from build123d import *

# Parameters (mm, degrees)
F0_W      = 60.442928
F0_H      = 76.316834
F1_DEPTH  = 13
F2_R      = 4.501425
F3_DEPTH  = 7.874
F4_R      = 3.44672
F5_DEPTH  = 16.764
F6_W      = 10
F6_H      = 4.021608
F7_DEPTH  = 0.7
F8_W      = 12.088504
F8_H      = 2.308511
F9_DEPTH  = 7.874
F10_W     = 10
F10_H     = 2.673487
F11_DEPTH = 8.636
F12_W     = 10.518157
F12_H     = 2.767401
F13_DEPTH = 29.718
F14_R     = 1.567214
F15_DEPTH = 1
F16_W     = 1.627309
F16_H     = 5.575751
F17_DEPTH = 1


with BuildPart() as f1:
    # F0 (on Front) → F1 (new body)
    with BuildSketch(Plane.XZ):
        Rectangle(F0_W, F0_H)
    extrude(amount=F1_DEPTH)

    # F2 (on face) → F3 (cut)
    with BuildSketch(Plane(origin=(0, 0, 0), x_dir=(-1, 0, 0), z_dir=(0, 1, 0))):
        with Locations((-20.47102, 49.871981)):
            Circle(F2_R)
    extrude(amount=F3_DEPTH, mode=Mode.SUBTRACT)

    # F4 (on face) → F5 (cut)
    with BuildSketch(Plane.XY.offset(38.158417)):
        with Locations((22.332672, -8.926389)):
            Circle(F4_R)
    extrude(amount=-F5_DEPTH, mode=Mode.SUBTRACT)

    # F6 (on face) → F7 (join)
    with BuildSketch(Plane(origin=(0, 0, -38.158417), x_dir=(1, 0, 0), z_dir=(0, 0, -1))):
        with Locations((-17.087876, 8.49799)):
            Rectangle(F6_W, F6_H)
    extrude(amount=F7_DEPTH)

    # F8 (on face) → F9 (join)
    with BuildSketch(Plane.XY.offset(38.158417)):
        with Locations((0.475428, -10.475016)):
            Rectangle(F8_W, F8_H)
    extrude(amount=-F9_DEPTH)

    # F10 (on face) → F11 (join)
    with BuildSketch(Plane.XY.offset(38.158417)):
        with Locations((-1.288279, -8.985477)):
            Rectangle(F10_W, F10_H)
    extrude(amount=-F11_DEPTH)

    # F12 (on face) → F13 (cut)
    with BuildSketch(Plane.XY.offset(38.158417)):
        with Locations((0.831678, -10.416227)):
            Rectangle(F12_W, F12_H)
    extrude(amount=-F13_DEPTH, mode=Mode.SUBTRACT)

    # F14 (on face) → F15 (join)
    with BuildSketch(Plane(origin=(-30.221464, 0, 0), x_dir=(0, -1, 0), z_dir=(-1, 0, 0))):
        with Locations((4.903499, -25.651673)):
            Circle(F14_R)
    extrude(amount=F15_DEPTH)

    # F16 (on face) → F17 (join)
    with BuildSketch(Plane(origin=(-30.221464, 0, 0), x_dir=(0, -1, 0), z_dir=(-1, 0, 0))):
        with Locations((4.771643, -18.09097)):
            Rectangle(F16_W, F16_H)
    extrude(amount=F17_DEPTH)


solid = f1.part
Could you check a few things on this model? Use its own coordinates, in mm. A direction names the side the tool comes from. Coordinates: 2 decimals unless noted, no trailing zeros. Order: outer loops, then holes, each group sorted by start corner. A loop starts at its lowest first (then second) coordinate and runs counter-clockwise, first axis right, second up.
Q1. Please list where these lines run through material, in increasing order: L1, parallel to Y at x = -2, z = 10; L2, parallel to Z at x = -27.5, y = -10.75; L3, parallel to X at y = -3.5, z = 30.
Q2. Will these pins go through, and if not, where does the flat tip stop? pin 1 (0.8 mm diameter, centred on x = -30.5, z = -19, fed in from +Y); pin 2 (1 mm diameter, centred on x = -2, y = -3.5, fed in from -Z); pin 3 (2 mm diameter, centred on x = -0.5, y = -10.5, fed in from +Z); pin 4 (0.5 mm diameter, centred on x = -31, y = -5, fed in from -Z).
Q3. Suppose I cut it at C-C on z = 29.5. Please give me the cut outline in (x, y), and give its area (3 significant figures).
Q4. Which directions (+Z, -Z, +X, -X, +Y, -Y) give clear straight access to the entire face, cutting with the end or side of a thin tool? Please do faces 1 (the flat face through (22, -9, 21.394)), 2 (the flat face through (-31.221, -5, -26)), 3 (the cylindrical face through (-30.71, -4.56, -27.18)).
Q5. Suppose I cut it at B-B on x = -0.5. Please give me the cut outline in (y, z), and give its area (3 significant figures).
Q6. Suppose I cut it at A-A on z = 12.5. Please give me the cut outline in (x, y).
Q7. Suppose I cut it at D-D on y = -7.75. Please give me the cut outline in (x, z).
Answer:
1. L1: y = -13 to -11.8, -9.03 to 0
1. L2: z = -38.16 to 38.16
1. L3: x = -30.22 to 30.22
2. pin 1: stops at y = 0
2. pin 2: stops at z = -38.16
2. pin 3: stops at z = 8.44
2. pin 4: stops at z = -27.22
3. outline: (-30.22, -13) - (30.22, -13) - (30.22, 0) - (-30.22, 0) - close; hole (-4.43, -11.8) - (6.09, -11.8) - (6.09, -9.03) - (-4.43, -9.03) - close; hole circle Ø6.89 at (22.33, -8.93)
3. area: 719 mm2
4. face 1: +Z
4. face 2: +Z, -Z, -X, +Y, -Y
4. face 3: -X
5. outline: (-13, -38.16) - (0, -38.16) - (0, 38.16) - (-9.03, 38.16) - (-9.03, 8.44) - (-11.8, 8.44) - (-11.8, 38.16) - (-13, 38.16) - close
5. area: 910 mm2
6. outline: (-30.22, -13) - (30.22, -13) - (30.22, 0) - (-30.22, 0) - close; hole (-4.43, -11.8) - (6.09, -11.8) - (6.09, -9.03) - (-4.43, -9.03) - close
7. outline: (-30.22, -38.16) - (-22.09, -38.16) - (-22.09, -38.86) - (-12.09, -38.86) - (-12.09, -38.16) - (30.22, -38.16) - (30.22, 38.16) - (25.57, 38.16) - (25.57, 21.39) - (19.09, 21.39) - (19.09, 38.16) - (-30.22, 38.16) - close
